Design review of the part built by this model. Coordinates are the model's own, in mm. A direction names the side the tool comes from. Round coordinates to 2 decimals unless told otherwise and drop trailing zeros. Write each loop counter-clockwise with the first axis right and the second up, starting at its lowest first coordinate (ties: lowest second). Pieces come first, ordered by that corner, then holes. Notation, with made-up numbers: (38, 53) -> (90, 53) arc R13 cw to (90, 74) -> close; hole circle Ø10 at (16.5, 79). An arc over 180 degrees is marked (long way). One line per question, with ' | ' between items. Start each with the question number.
1) Consider section B-B (x = 12.5). Give the boundary of the cut face in (y, z).
2) Consider section A-A (z = -7). Give the boundary of the cut face in (x, y), then the cut area to 3 significant figures.
3) Consider section C-C (y = 27.5). Give the boundary of the cut face in (x, z).
4) Consider section D-D (z = -25). Give the boundary of the cut face in (x, y), then the cut area to 3 significant figures.
5) Mouldability with a two-part tool opening along Y and no side actions: class faces 1 (the flat face through (12, 8, -6)), 2 (the flat face through (12, 18, -48)), 3 (the cylindrical face through (0.43, 37.55, -25.33)), 4 (the flat face through (1, 9, -30)) as +Y half, -Y half, draft (parallel to the pull), parting line (faces both ways), or undercut.
6) For probe 1 along Y at (x, z) = (12.5, -7); probe 2 along Z at (x, y) = (5, 34); probe 3 along X at (y, z) = (20, -33), list the stretches that pass through material, from the lowest coordinate up.
7) For faces 5 (the flat face through (4.5, 12, -6)), 6 (the cylindrical face through (28.9, 2.4, -26.2)), 7 (the flat face through (12, 38, -25)), 8 (the flat face through (1, 4, -38)), 9 (the flat face through (12, 0, -12)), list the 3-axis set-ups (+Z, -Z, +X, -X, +Y, -Y) from which the entire face can be reached by the end or side of a thin tool; tool diameter is ignored.
8) Insertion check: pin 1 Ø6.5 at (x, z) = (12, -37) entering from -Y; pin 2 Ø10 at (y, z) = (14, -8) entering from +X; pin 3 Ø3 at (x, y) = (14, 11.5) entering from +Z. Each pin has a flat end and moves straight along its axis. Give the tip position at first contact, or say it passes through.
```python
from build123d import *

# Parameters (mm, degrees)
SKETCH_1_W          = 25
SKETCH_1_H          = 38
EXTRUDE_1_DEPTH     = 50
SKETCH_2_R          = 7.5
CUT_EXTRUDE_1_DEPTH = 13
SKETCH_3_W          = 21
SKETCH_3_H          = 36
CUT_EXTRUDE_2_DEPTH = 35
SKETCH_4_W          = 16
SKETCH_4_H          = 9
CUT_EXTRUDE_3_DEPTH = 10
FILLET_1_R          = 1.5
FILLET_2_R          = 1.5
FILLET_3_R          = 1.5
SKETCH_5_R          = 2
EXTRUDE_2_DEPTH     = 8
CUT_EXTRUDE_4_REACH = 72.944
SKETCH_6_W          = 16
SKETCH_6_H          = 9


with BuildPart() as part:
    # 草图1 → 凸台-拉伸1 (new body)
    with BuildSketch(Plane.XY):
        with Locations((12.5, 19)):
            Rectangle(SKETCH_1_W, SKETCH_1_H)
    extrude(amount=-EXTRUDE_1_DEPTH)

    # 草图2 → 切除-拉伸1 (cut)
    with BuildSketch(Plane.XY):
        with Locations((12.5, 27.5)):
            Circle(SKETCH_2_R)
    extrude(amount=-CUT_EXTRUDE_1_DEPTH, mode=Mode.SUBTRACT)

    # 草图3 → 切除-拉伸2 (cut)
    with BuildSketch(Plane.XY.offset(-13)):
        with Locations((12.5, 18)):
            Rectangle(SKETCH_3_W, SKETCH_3_H)
    extrude(amount=-CUT_EXTRUDE_2_DEPTH, mode=Mode.SUBTRACT)

    # 草图4 → 切除-拉伸3 (cut)
    with BuildSketch(Plane(origin=(2, 0, 0), x_dir=(0, 0, -1), z_dir=(1, 0, 0))):
        with Locations((30, 4.5)):
            Rectangle(SKETCH_4_W, SKETCH_4_H)
    extrude(amount=-CUT_EXTRUDE_3_DEPTH, mode=Mode.SUBTRACT)

    # 圆角1
    fillet_1_edges = [part.edges().sort_by_distance(p)[0] for p in [
        (12.5, 38, -50),
        (12.5, 38, 0),
        (0, 38, -25),
        (25, 38, -25),
    ]]
    fillet(fillet_1_edges, radius=FILLET_1_R)

    # 圆角2
    # the kernel refuses this fillet: 1.5 mm, written as the material it takes off along each edge
    with BuildSketch(Plane(origin=(1.5, 36.5, -48.5), x_dir=(0, 0, -1), z_dir=(-1, 0, 0))) as fillet_2_piece_1_section:
        Polygon((0, 0), (FILLET_2_R, 0), (FILLET_2_R, -FILLET_2_R), (0, -FILLET_2_R), align=None)
    fillet_2_piece_1 = extrude(amount=FILLET_2_R, mode=Mode.PRIVATE)
    fillet_2_piece_1 = fillet_2_piece_1 - Plane(origin=(1.5, 36.5, -48.5), x_dir=(0, -0.7071067811865475, 0.7071067811865475), z_dir=(-1, 0, 0)) * Sphere(FILLET_2_R, mode=Mode.PRIVATE)
    add(fillet_2_piece_1, mode=Mode.SUBTRACT)
    with BuildSketch(Plane(origin=(1.5, 36.5, -1.5), x_dir=(0, 0, 1), z_dir=(-1, 0, 0))) as fillet_2_piece_2_section:
        Polygon((0, 0), (FILLET_2_R, 0), (FILLET_2_R, FILLET_2_R), (0, FILLET_2_R), align=None)
    fillet_2_piece_2 = extrude(amount=FILLET_2_R, mode=Mode.PRIVATE)
    fillet_2_piece_2 = fillet_2_piece_2 - Plane(origin=(1.5, 36.5, -1.5), x_dir=(0, -0.7071067811865475, -0.7071067811865475), z_dir=(-1, 0, 0)) * Sphere(FILLET_2_R, mode=Mode.PRIVATE)
    add(fillet_2_piece_2, mode=Mode.SUBTRACT)
    with BuildSketch(Plane(origin=(23.5, 36.5, -48.5), x_dir=(1, 0, 0), z_dir=(0, 0, -1))) as fillet_2_piece_3_section:
        Polygon((0, 0), (FILLET_2_R, 0), (FILLET_2_R, -FILLET_2_R), (0, -FILLET_2_R), align=None)
    fillet_2_piece_3 = extrude(amount=FILLET_2_R, mode=Mode.PRIVATE)
    fillet_2_piece_3 = fillet_2_piece_3 - Plane(origin=(23.5, 36.5, -48.5), x_dir=(-0.7071067811865476, -0.7071067811865476, 0), z_dir=(0, 0, -1)) * Sphere(FILLET_2_R, mode=Mode.PRIVATE)
    add(fillet_2_piece_3, mode=Mode.SUBTRACT)
    with BuildSketch(Plane(origin=(0, -3.75, -50), x_dir=(0, 0, 1), z_dir=(0, 1, 0))) as fillet_2_piece_4:
        with BuildLine():
            CenterArc((FILLET_2_R, FILLET_2_R), FILLET_2_R, 180, 90)
            Line((0, FILLET_2_R), (0, 0))
            Line((0, 0), (FILLET_2_R, 0))
        make_face()
    extrude(amount=40.25, mode=Mode.SUBTRACT)
    with BuildSketch(Plane(origin=(0, -3.75, 0), x_dir=(0, 0, -1), z_dir=(0, 1, 0)), Plane(origin=(25, 36.5, -50), x_dir=(-1, 0, 0), z_dir=(0, -1, 0))) as fillet_2_piece_5:
        with BuildLine():
            CenterArc((FILLET_2_R, -FILLET_2_R), FILLET_2_R, 90, 90)
            Line((0, -FILLET_2_R), (0, 0))
            Line((0, 0), (FILLET_2_R, 0))
        make_face()
    extrude(amount=40.25, mode=Mode.SUBTRACT)

    # 圆角3
    # the kernel refuses this fillet: 1.5 mm, written as the material it takes off along each edge
    with BuildSketch(Plane(origin=(23.5, 36.5, -1.5), x_dir=(1, 0, 0), z_dir=(0, 0, 1))) as fillet_3_piece_1_section:
        Polygon((0, 0), (FILLET_3_R, 0), (FILLET_3_R, FILLET_3_R), (0, FILLET_3_R), align=None)
    fillet_3_piece_1 = extrude(amount=FILLET_3_R, mode=Mode.PRIVATE)
    fillet_3_piece_1 = fillet_3_piece_1 - Plane(origin=(23.5, 36.5, -1.5), x_dir=(-0.7071067811865476, -0.7071067811865476, 0), z_dir=(0, 0, 1)) * Sphere(FILLET_3_R, mode=Mode.PRIVATE)
    add(fillet_3_piece_1, mode=Mode.SUBTRACT)
    with BuildSketch(Plane(origin=(25, 36.5, 0), x_dir=(-1, 0, 0), z_dir=(0, -1, 0))) as fillet_3_piece_2:
        with BuildLine():
            CenterArc((FILLET_3_R, FILLET_3_R), FILLET_3_R, 180, 90)
            Line((0, FILLET_3_R), (0, 0))
            Line((0, 0), (FILLET_3_R, 0))
        make_face()
    extrude(amount=40.25, mode=Mode.SUBTRACT)

    # 草图5 → 凸台-拉伸2 (add)
    with BuildSketch(Plane(origin=(25, 0, 0), x_dir=(0, 0, -1), z_dir=(1, 0, 0))):
        with Locations(Location((25, 4, 0), (0, 0, 90))):
            Circle(SKETCH_5_R)
    extrude(amount=EXTRUDE_2_DEPTH)

    # 草图6 → 切除-拉伸4 (cut, up to next)
    with BuildSketch(Plane.XY, mode=Mode.PRIVATE) as cut_extrude_4_sk1:
        with Locations((12.5, 12.5)):
            Rectangle(SKETCH_6_W, SKETCH_6_H)
    cut_extrude_4_tool1 = extrude(cut_extrude_4_sk1.sketch, amount=-CUT_EXTRUDE_4_REACH, mode=Mode.PRIVATE) & part.part
    add(cut_extrude_4_tool1.solids().sort_by_distance((12.5, 12.5, 0))[0], mode=Mode.SUBTRACT)


solid = part.part
```
From the geometry:
1) outline: (0, -50) -> (36.5, -50) arc R1.5 ccw to (38, -48.5) -> (38, -1.5) arc R1.5 ccw to (36.5, 0) -> (35, 0) -> (35, -13) -> (36, -13) -> (36, -48) -> (0, -48) -> close; (0, -13) -> (8, -13) -> (8, 0) -> (0, 0) -> close; (17, -13) -> (20, -13) -> (20, 0) -> (17, 0) -> close
2) outline: (0, 0) -> (25, 0) -> (25, 36.5) arc R1.5 ccw to (23.5, 38) -> (1.5, 38) arc R1.5 ccw to (0, 36.5) -> close; hole (4.5, 8) -> (20.5, 8) -> (20.5, 17) -> (4.5, 17) -> close; hole circle Ø15 at (12.5, 27.5) | area: 628 mm2
3) outline: (0, -48.5) arc R1.5 ccw to (1.5, -50) -> (23.5, -50) arc R1.5 ccw to (25, -48.5) -> (25, -1.5) arc R1.5 ccw to (23.5, 0) -> (20, 0) -> (20, -13) -> (23, -13) -> (23, -48) -> (2, -48) -> (2, -13) -> (5, -13) -> (5, 0) -> (1.5, 0) arc R1.5 ccw to (0, -1.5) -> close
4) outline: (0, 9) -> (2, 9) -> (2, 36) -> (23, 36) -> (23, 0) -> (25, 0) -> (25, 2) -> (33, 2) -> (33, 6) -> (25, 6) -> (25, 36.5) arc R1.5 ccw to (23.5, 38) -> (1.5, 38) arc R1.5 ccw to (0, 36.5) -> close | area: 207 mm2
5) face 1: undercut | face 2: draft | face 3: +Y half | face 4: -Y half
6) probe 1: y = 0 to 8, 17 to 20, 35 to 38 | probe 2: z = -50 to -48, -13 to 0 | probe 3: x = 0 to 2, 23 to 25
7) face 5: +Z | face 6: +X | face 7: +Z, -Z, +X, -X, +Y | face 8: -X, -Y | face 9: +Z, -Z, +X, -X, -Y
8) pin 1: stops at y = 36 | pin 2: stops at x = 25 | pin 3: stops at z = -48
